```python
from build123d import *

# Parameters (mm, degrees)
EXTRUDE1_DEPTH = 6


with BuildPart() as part:
    # Sketch1 → Extrude1 (new body)
    with BuildSketch(Plane.XY):
        with BuildLine():
            Line((-9.389431256, -4.992449157), (-84.389431256, -44.870656531))
            ThreePointArc((-84.389431256, -44.870656531), (-92.143346014, -52.22884689), (-95, -62.529608388))
            Line((-95, -62.529608388), (-95, -81.512396008))
            ThreePointArc((-95, -81.512396008), (-95.878679656, -83.633716351), (-98, -84.512396008))
            Line((-98, -84.512396008), (-112, -84.512396008))
            ThreePointArc((-112, -84.512396008), (-114.121320344, -83.633716351), (-115, -81.512396008))
            Line((-115, -81.512396008), (-115, -40.567908762))
            ThreePointArc((-115, -40.567908762), (-114.14184053, -34.772225789), (-111.641005887, -29.473904838))
            Line((-111.641005887, -29.473904838), (-58.358994113, 50.449112822))
            ThreePointArc((-58.358994113, 50.449112822), (-55.85815947, 55.747433773), (-55, 61.543116747))
            Line((-55, 61.543116747), (-55, 67.487603992))
            ThreePointArc((-55, 67.487603992), (-54.121320344, 69.608924336), (-52, 70.487603992))
            Line((-52, 70.487603992), (-28.840084091, 70.487603992))
            ThreePointArc((-28.840084091, 70.487603992), (-26.834640517, 69.718791136), (-25.85707081, 67.806401373))
            add(Edge.make_bspline(
                [(-25.85707081, 67.806401373), (-23.204663037, 42.987603992), (4, 42.987603992), (31.204663037, 42.987603992), (33.85707081, 67.806401373)],
                knots=[3.239246064, 3.239246064, 3.239246064, 4.71238898, 4.71238898, 6.185531897, 6.185531897, 6.185531897], degree=2, weights=[1, 0.740776038, 1, 0.740776038, 1]))
            ThreePointArc((33.85707081, 67.806401373), (34.834640517, 69.718791136), (36.840084091, 70.487603992))
            Line((36.840084091, 70.487603992), (69, 70.487603992))
            ThreePointArc((69, 70.487603992), (71.121320344, 69.608924336), (72, 67.487603992))
            Line((72, 67.487603992), (72, 17.487603992))
            ThreePointArc((72, 17.487603992), (73.464466094, 13.952070086), (77, 12.487603992))
            Line((77, 12.487603992), (174, 12.487603992))
            ThreePointArc((174, 12.487603992), (176.121320344, 11.608924336), (177, 9.487603992))
            Line((177, 9.487603992), (177, -16.208108765))
            ThreePointArc((177, -16.208108765), (175.834161378, -20.894001715), (172.608481452, -24.48729567))
            Line((172.608481452, -24.48729567), (123.783037097, -57.562596684))
            ThreePointArc((123.783037097, -57.562596684), (117.331677243, -64.749184594), (115, -74.120970494))
            Line((115, -74.120970494), (115, -81.512396008))
            ThreePointArc((115, -81.512396008), (114.121320344, -83.633716351), (112, -84.512396008))
            Line((112, -84.512396008), (98, -84.512396008))
            ThreePointArc((98, -84.512396008), (95.878679656, -83.633716351), (95, -81.512396008))
            Line((95, -81.512396008), (95, -62.529608388))
            ThreePointArc((95, -62.529608388), (92.143346014, -52.22884689), (84.389431256, -44.870656531))
            Line((84.389431256, -44.870656531), (9.389431256, -4.992449157))
            ThreePointArc((9.389431256, -4.992449157), (0, -2.651401014), (-9.389431256, -4.992449157))
        make_face()
    extrude(amount=EXTRUDE1_DEPTH)


solid = part.part
```
Build history of the part. All positions in model axes, mm. A direction names the side the tool comes from. Coordinates: 2 decimals unless noted, no trailing zeros. Order: outer loops, then holes, each group sorted by start corner. A loop starts at its lowest first (then second) coordinate and runs counter-clockwise, first axis right, second up. Notation, with made-up numbers: (74.5, 17.5) -> (113.5, 17.5) arc R28 ccw to (113.5, 44.5) -> close; hole circle Ø3 at (66, 2.25). An arc over 180 degrees is marked (long way). Answer in a Markdown table with one row per item. Add a question column.
Q1. Drop flat-ended pins along their axis: pin 1 (3 mm diameter, centred on y = 31.5, z = 2, fed in from +X); pin 2 (3 mm diameter, centred on x = 126.5, z = 0.5, fed in from -Y); pin 3 (3 mm diameter, centred on x = 135, z = 3, fed in from +Y). Give the stop position or say it passes through.
Q2. Mould opens along X. For faces 6 (the face through (-114.166, -34.851, 2.958)), 7 (the face through (-46.36, -24.65, 2.96)), 8 (the face through (47.41, -25.21, 2.96)), 9 (the face through (-41, 70.488, 3)) say: +X half, -X half, draft (parallel to the pull), parting line (faces both ways), or undercut.
Q3. Band-saw the part on B-B, the plane y = 29.5. List the corners of the cut face in (x, z), then the cut area to 3 significant figures.
Q4. Band-saw the part on A-A, the plane x = -41.5. List the corners of the cut face in (y, z), then the cut area to 3 significant figures.
Q5. Which spindle directions (+Z, -Z, +X, -X, +Y, -Y) get a long thin tool onto all of the face, cutting with end or side? Do faces 1 (the face through (177, -3, 3)), 2 (the face through (115, -78, 3)), 3 (the face through (95, -72, 3)), 4 (the face through (-105, -84.512, 3)), 5 (the face through (-55, 64, 3)). Say none if no direction does.
Q6. Wall check: line 1 along X through (y, z) = (-12, 5.75); line 2 along X through (y, z) = (-68, 4.75); line 3 along Y through (x, z) = (127.5, 0.5). Give the ranges that are in metal, low to high. Write a range as [from, to].
Answers follow:
| question | item | result |
|---|---|---|
| 1 | pin 1 | x = 72 |
| 1 | pin 2 | y = -56.74 |
| 1 | pin 3 | y = 12.49 |
| 2 | face 6 | -X half |
| 2 | face 7 | undercut |
| 2 | face 8 | undercut |
| 2 | face 9 | draft |
| 3 | outline | (-72.33, 0) -> (72, 0) -> (72, 6) -> (-72.33, 6) -> close |
| 3 | area | 866 mm^2 |
| 4 | outline | (-22.07, 0) -> (70.49, 0) -> (70.49, 6) -> (-22.07, 6) -> close |
| 4 | area | 555 mm^2 |
| 5 | face 1 | +Z, -Z, +X, +Y, -Y |
| 5 | face 2 | +Z, -Z, +X, -Y |
| 5 | face 3 | +Z, -Z, -Y |
| 5 | face 4 | +Z, -Z, +X, -X, -Y |
| 5 | face 5 | +Z, -Z, -X, +Y |
| 6 | line 1 | [-99.99, -22.57], [22.57, 177] |
| 6 | line 2 | [-115, -95], [95, 115.96] |
| 6 | line 3 | [-55.04, 12.49] |
